Check sheet for the modelled part. Datum: model origin and axes. Units: mm. Face numbers are marked on the shaded views. A direction names the side the tool comes from. Give positions to 0.01 mm unless a question says otherwise; leave off trailing zeros. Order: outer loops, then holes, each group sorted by start corner. A loop starts at its lowest first (then second) coordinate and runs counter-clockwise, first axis right, second up.
```python
from build123d import *

# Parameters (mm, degrees)
ESQUISSE2_R             = 2.1
BOSS_EXTRU_1_DEPTH      = 5
ESQUISSE4_R             = 2.1
BOSS_EXTRU_2_DEPTH      = 3
ESQUISSE6_R             = 1.1
ENL_V_MAT_EXTRU_1_DEPTH = 10


with BuildPart() as part:
    # Esquisse2 → Boss.-Extru.1 (new body)
    with BuildSketch(Plane.XY):
        with BuildLine():
            Line((18, 0.75), (-13, 0.75))
            ThreePointArc((-13, 0.75), (-14.414213562, 0.164213562), (-15, -1.25))
            Line((-15, -1.25), (-15, -12.25))
            ThreePointArc((-15, -12.25), (-14.414213562, -13.664213562), (-13, -14.25))
            Line((-13, -14.25), (18, -14.25))
            ThreePointArc((18, -14.25), (19.414213562, -13.664213562), (20, -12.25))
            Line((20, -12.25), (20, -1.25))
            ThreePointArc((20, -1.25), (19.414213562, 0.164213562), (18, 0.75))
        make_face()
        with Locations((-8, -10.25)):
            Circle(ESQUISSE2_R, mode=Mode.SUBTRACT)
        with Locations((-8, -3.25)):
            Circle(ESQUISSE2_R, mode=Mode.SUBTRACT)
    extrude(amount=BOSS_EXTRU_1_DEPTH)

    # Esquisse4 → Boss.-Extru.2 (add)
    with BuildSketch(Plane.XY.offset(5)):
        with BuildLine():
            Line((0, 0.75), (0, -14.25))
            Line((0, -14.25), (-13, -14.25))
            ThreePointArc((-13, -14.25), (-14.414213562, -13.664213562), (-15, -12.25))
            Line((-15, -12.25), (-15, -1.25))
            ThreePointArc((-15, -1.25), (-14.414213562, 0.164213562), (-13, 0.75))
            Line((-13, 0.75), (0, 0.75))
        make_face()
        with Locations((-8, -10.25)):
            Circle(ESQUISSE4_R, mode=Mode.SUBTRACT)
        with Locations((-8, -3.25)):
            Circle(ESQUISSE4_R, mode=Mode.SUBTRACT)
    extrude(amount=BOSS_EXTRU_2_DEPTH)

    # Esquisse6 → Enlèv. mat.-Extru.1 (cut)
    with BuildSketch(Plane(origin=(0, 0, 0), x_dir=(-1, 0, 0), z_dir=(0, 0, -1))):
        with Locations((-15, -7.997523441)):
            Circle(ESQUISSE6_R)
        with BuildLine():
            Line((-5.249999883, -6.914758131), (-4.478449657, -6.914758131))
            ThreePointArc((-4.478449657, -6.914758131), (-3.393207978, -7.99999981), (-4.478449657, -9.085241489))
            Line((-4.478449657, -9.085241489), (-5.249999883, -9.085241489))
            ThreePointArc((-5.249999883, -9.085241489), (-6.335241562, -7.99999981), (-5.249999883, -6.914758131))
        make_face()
    extrude(amount=-ENL_V_MAT_EXTRU_1_DEPTH, mode=Mode.SUBTRACT)


solid = part.part
```
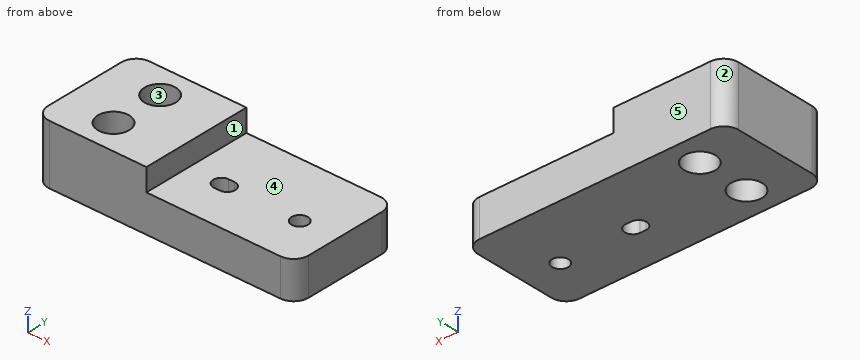
(1) Cross-section at C-C on y = -10.25. Enter the section's corners in (x, z), then the cut area to 3 significant figures.
Response values:
outline: (-15, 0) - (-10.1, 0) - (-10.1, 8) - (-15, 8) - close; (-5.9, 0) - (20, 0) - (20, 5) - (0, 5) - (0, 8) - (-5.9, 8) - close
area: 186 mm2
(2) Material ranges on L1, parallel to Y at x = -8, z = 5.5; L2, parallel to Z at x = 10, y = -12.5; L3, parallel to Y at x = 4.5, z = 2.75, recorded low to high.
Response values:
L1: y = -14.25 to -12.35, -8.15 to -5.35, -1.15 to 0.75
L2: z = 0 to 5
L3: y = -14.25 to -9.09, -6.91 to 0.75
(3) Gauge pin test, flat ends, axial feed: pin 1 Ø4.5 at (x, y) = (12, -6) entering from +Z; pin 2 Ø2.5 at (y, z) = (-10.5, 7) entering from +X. Record the tip position at first contact, or that the pin passes through.
Response values:
pin 1: stops at z = 5
pin 2: stops at x = 0
(4) Cross-section at D-D on x = -8. Enter the section's corners in (y, z).
Response values:
outline: (-14.25, 0) - (-12.35, 0) - (-12.35, 8) - (-14.25, 8) - close; (-8.15, 0) - (-5.35, 0) - (-5.35, 8) - (-8.15, 8) - close; (-1.15, 0) - (0.75, 0) - (0.75, 8) - (-1.15, 8) - close
(5) Cross-section at B-B on z = 6. Enter the section's corners in (x, y), then the cut area to 3 significant figures.
Response values:
outline: (-15, -12.25) arc R2 ccw to (-13, -14.25) - (0, -14.25) - (0, 0.75) - (-13, 0.75) arc R2 ccw to (-15, -1.25) - close; hole circle Ø4.2 at (-8, -10.25); hole circle Ø4.2 at (-8, -3.25)
area: 196 mm2
(6) Release check for a two-part mould opening along Y. For the marked faces 3, 4 and 5 record: released by +Y, released by -Y, zero draft, split by the parting line, or undercut.
Response values:
face 3: undercut
face 4: zero draft
face 5: released by +Y
(7) Cross-section at A-A on x = 15. Enter the section's corners in (y, z).
Response values:
outline: (-14.25, 0) - (-9.1, 0) - (-9.1, 5) - (-14.25, 5) - close; (-6.9, 0) - (0.75, 0) - (0.75, 5) - (-6.9, 5) - close
(8) Set-up check for the marked faces 1 and 2: record each of +Z, -Z, +X, -X, +Y, -Y from which the full face is reachable in a straight line by a thin tool's end or side.
Response values:
face 1: +Z, +X, +Y, -Y
face 2: +Z, -Z, -X, +Y
